Part print with two shaded views. Sizes in mm from the minimum x, y, z corner. A direction names the side the tool comes from. Coordinates: 2 decimals unless noted, no trailing zeros. Loops run counter-clockwise (first coordinate to the right, second up) from the corner with the lowest first, then second, coordinate; pieces in that order, holes last.
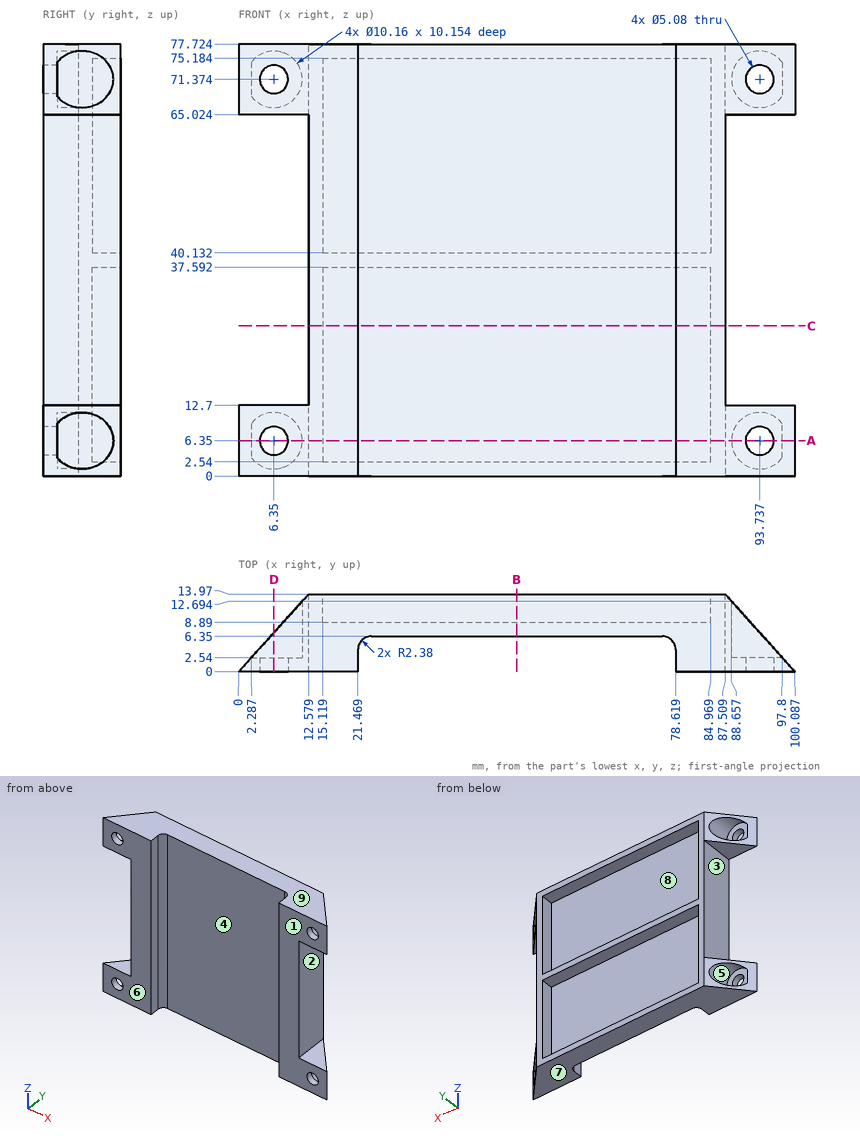
Q1. Mould opens along Z. For the marked faces 6, 7, 8 and 9 say: +Z half, -Z half, draft (parallel to the pull), parting line (faces both ways), or undercut.
Answers:
face 6: draft
face 7: -Z half
face 8: undercut
face 9: +Z half
Q2. Slice it at D-D (x = 6.35). List the corners of the cut face in (y, z).
Answers:
outline: (0, 0) - (7.05, 0) - (7.05, 1.27) - (2.54, 1.27) - (2.54, 3.81) - (0, 3.81) - close; (0, 8.89) - (2.54, 8.89) - (2.54, 11.43) - (7.05, 11.43) - (7.05, 12.7) - (0, 12.7) - close; (0, 65.02) - (7.05, 65.02) - (7.05, 66.29) - (2.54, 66.29) - (2.54, 68.83) - (0, 68.83) - close; (0, 73.91) - (2.54, 73.91) - (2.54, 76.45) - (7.05, 76.45) - (7.05, 77.72) - (0, 77.72) - close
Q3. Which spindle directions (+Z, -Z, +X, -X, +Y, -Y) get a long thin tool onto all of the face, cutting with end or side? Do the marked faces 1, 2, 3, 4 and 5. Say none if no direction does.
Answers:
face 1: +Z, -Z, +X, -X, -Y
face 2: +X, +Y, -Y
face 3: -X, +Y, -Y
face 4: +Z, -Z, -Y
face 5: +Y
Q4. Flat gauge pins, fed straight in: P1, Ø8, axis at x = 74, z = 62, coming from the -Y side; P2, Ø6, axis at x = 41, z = 11.5, coming from the +Y side; P3, Ø2.5, axis at x = 5.5, z = 69.5, coming from the +Y side; P4, Ø3, axis at x = 27.5, y = 5.5, coming from the -Z side. Where does each tip first touch, or does it go through?
Answers:
P1: stops at y = 5.57
P2: stops at y = 8.89
P3: stops at y = 2.54
P4: stops at z = 0
Q5. Drill centre lines: line 1 (Z direction, x = 82, y = 12.5); line 2 (X direction, y = 1.5, z = 58.5); line 3 (Z direction, x = 6.35, y = 0.85). Where is each one in solid material? Low to high.
Answers:
line 1: z = 0 to 2.54, 37.59 to 40.13, 75.18 to 77.72
line 2: x = 12.58 to 21.47, 78.62 to 87.51
line 3: z = 0 to 3.81, 8.89 to 12.7, 65.02 to 68.83, 73.91 to 77.72
Q6. Slice it at A-A (z = 6.35). Count the separate pieces of the cut face and the enclosed holes in it.
Answers:
separate pieces: 3
enclosed holes: 0
Q7. Slice it at C-C (z = 27). List the corners of the cut face in (x, y).
Answers:
outline: (12.58, 0) - (21.47, 0) - (21.47, 3.97) arc R2.38 cw to (23.85, 6.35) - (76.24, 6.35) arc R2.38 cw to (78.62, 3.97) - (78.62, 0) - (87.51, 0) - (87.51, 13.97) - (84.97, 13.97) - (84.97, 8.89) - (15.12, 8.89) - (15.12, 13.97) - (12.58, 13.97) - close
Q8. Slice it at B-B (x = 50). List the corners of the cut face in (y, z), and give its area (3 significant figures).
Answers:
outline: (6.35, 0) - (13.97, 0) - (13.97, 2.54) - (8.89, 2.54) - (8.89, 37.59) - (13.97, 37.59) - (13.97, 40.13) - (8.89, 40.13) - (8.89, 75.18) - (13.97, 75.18) - (13.97, 77.72) - (6.35, 77.72) - close
area: 236 mm2
